```python
from build123d import *

# Parameters (mm, degrees)
SKETCH1_R           = 79.480373192
BOSS_EXTRUDE1_DEPTH = 10
BOSS_EXTRUDE2_DEPTH = 70
FILLET3_R           = 5
SKETCH7_R           = 2.5
CUT_EXTRUDE4_DEPTH  = 138.964703622
CUT_EXTRUDE6_DEPTH  = 2.5
FILLET5_RADIUS      = 20
FILLET5_LENGTH      = 10
CUT_EXTRUDE7_DEPTH  = 2.5


with BuildPart() as part:
    # Sketch1 → Boss-Extrude1 (new body)
    with BuildSketch(Plane.XY):
        Circle(SKETCH1_R)
    extrude(amount=BOSS_EXTRUDE1_DEPTH)

    # Sketch2 → Boss-Extrude2 (add)
    with BuildSketch(Plane.XY.offset(10)):
        Polygon((0, 0), (0, -20), (-10, -20), (-10, 20), (0, 20), align=None)
    extrude(amount=BOSS_EXTRUDE2_DEPTH)

    # Fillet3
    fillet3_edges = [part.edges().sort_by_distance(p)[0] for p in [
        (-5, 20, 10),
        (-10, 0, 10),
        (-5, -20, 10),
        (0, 0, 10),
    ]]
    fillet(fillet3_edges, radius=FILLET3_R)

    # Sketch7 → Cut-Extrude4 (cut, through all)
    with BuildSketch(Plane(origin=(0, 0, 0), x_dir=(0, 0, -1), z_dir=(1, 0, 0))):
        with Locations(Location((-60, 0, 0), (0, 0, 90))):
            Circle(SKETCH7_R)
    extrude(amount=-CUT_EXTRUDE4_DEPTH, mode=Mode.SUBTRACT)

    # Sketch9 → Cut-Extrude6 (cut)
    with BuildSketch(Plane(origin=(0, 0, 0), x_dir=(0, 0, -1), z_dir=(1, 0, 0))):
        with BuildLine():
            Line((-64.239646316, 13.566264372), (-64.768269058, 6.229526416))
            Line((-64.768269058, 6.229526416), (-71.988493293, 7.63506113))
            ThreePointArc((-71.988493293, 7.63506113), (-74.774746239, 6.140592282), (-73.868552739, 3.111490773))
            Line((-73.868552739, 3.111490773), (-67.779062658, -1.014678928))
            Line((-67.779062658, -1.014678928), (-72.606403544, -6.56480918))
            ThreePointArc((-72.606403544, -6.56480918), (-72.70528203, -9.725009436), (-69.628906423, -10.454773599))
            Line((-69.628906423, -10.454773599), (-63.010793601, -7.244205344))
            Line((-63.010793601, -7.244205344), (-60.617910251, -14.19987031))
            ThreePointArc((-60.617910251, -14.19987031), (-57.930535791, -15.865601718), (-55.760353684, -13.566264372))
            Line((-55.760353684, -13.566264372), (-55.231730942, -6.229526416))
            Line((-55.231730942, -6.229526416), (-48.011506707, -7.63506113))
            ThreePointArc((-48.011506707, -7.63506113), (-45.225253761, -6.140592282), (-46.131447261, -3.111490773))
            Line((-46.131447261, -3.111490773), (-52.220937342, 1.014678928))
            Line((-52.220937342, 1.014678928), (-47.393596456, 6.56480918))
            ThreePointArc((-47.393596456, 6.56480918), (-47.29471797, 9.725009436), (-50.371093577, 10.454773599))
            Line((-50.371093577, 10.454773599), (-56.989206399, 7.244205344))
            Line((-56.989206399, 7.244205344), (-59.382089749, 14.19987031))
            ThreePointArc((-59.382089749, 14.19987031), (-62.069464209, 15.865601718), (-64.239646316, 13.566264372))
        make_face()
    extrude(amount=-CUT_EXTRUDE6_DEPTH, mode=Mode.SUBTRACT)

    # Fillet5: full round fillet: the end face becomes a half cylinder, R = half its width
    fillet5_face = Plane((-5, 0, 80), x_dir=(-1, 0, 0), z_dir=(0, 0, 1))  # on the end face: x along it, z out of the body
    fillet5_slab = fillet5_face.offset(-FILLET5_RADIUS / 2) * Box(FILLET5_LENGTH, 2 * FILLET5_RADIUS, FILLET5_RADIUS, mode=Mode.PRIVATE)  # the body's end, R deep
    fillet5_round = Plane((-5, 0, 60), x_dir=(0, 0, 1), z_dir=(-1, 0, 0)) * Cylinder(FILLET5_RADIUS, FILLET5_LENGTH, mode=Mode.PRIVATE)  # its axis R under the face
    add(fillet5_slab - fillet5_round, mode=Mode.SUBTRACT)

    # Sketch4 → Cut-Extrude7 (cut)
    with BuildSketch(Plane(origin=(0, 0, 0), x_dir=(-1, 0, 0), z_dir=(0, 0, -1))):
        with BuildLine():
            Line((-9.121537298, 10.900260879), (-6.793934197, 3.922479738))
            Line((-6.793934197, 3.922479738), (-14.000671478, 2.449352582))
            ThreePointArc((-14.000671478, 2.449352582), (-16, 0), (-14.000671478, -2.449352582))
            Line((-14.000671478, -2.449352582), (-6.793934197, -3.922479738))
            Line((-6.793934197, -3.922479738), (-9.121537298, -10.900260879))
            ThreePointArc((-9.121537298, -10.900260879), (-8, -13.856406461), (-4.87913418, -13.349613461))
            Line((-4.87913418, -13.349613461), (0, -7.844959475))
            Line((0, -7.844959475), (4.87913418, -13.349613461))
            ThreePointArc((4.87913418, -13.349613461), (8, -13.856406461), (9.121537298, -10.900260879))
            Line((9.121537298, -10.900260879), (6.793934197, -3.922479738))
            Line((6.793934197, -3.922479738), (14.000671478, -2.449352582))
            ThreePointArc((14.000671478, -2.449352582), (16, 0), (14.000671478, 2.449352582))
            Line((14.000671478, 2.449352582), (6.793934197, 3.922479738))
            Line((6.793934197, 3.922479738), (9.121537298, 10.900260879))
            ThreePointArc((9.121537298, 10.900260879), (8, 13.856406461), (4.87913418, 13.349613461))
            Line((4.87913418, 13.349613461), (0, 7.844959475))
            Line((0, 7.844959475), (-4.87913418, 13.349613461))
            ThreePointArc((-4.87913418, 13.349613461), (-8, 13.856406461), (-9.121537298, 10.900260879))
        make_face()
    extrude(amount=-CUT_EXTRUDE7_DEPTH, mode=Mode.SUBTRACT)


solid = part.part
```
Part model, mm, in its own coordinate system. A direction names the side the tool comes from. Round coordinates to 2 decimals unless told otherwise and drop trailing zeros. Order: outer loops, then holes, each group sorted by start corner. A loop starts at its lowest first (then second) coordinate and runs counter-clockwise, first axis right, second up. Notation, with made-up numbers: M -10,-6 L 3,-6 A24 ccw 3,31 Z; hole C 0.25,16.25 d9. An arc over 180 degrees is marked long. Answer in a Markdown table with one row per item. Add a question column.
Q1. Wall check: L1, parallel to Z at x = -6.75, y = 0; L2, parallel to Y at x = -1.5, z = 51.5; L3, parallel to X at y = -19, z = 22.5. Give the ranges that are in metal, low to high. Write a range as from..to.
Q2. 3-axis set-ups, long thin cutter, end or side, ignore diameter. For faces 1 (the face through (-2.474, 10.636, 1.232)), 2 (the face through (-5, -20, 37)), 3 (the face through (-1.2, -3.8, 70.2)): which of +Z, -Z, +X, -X, +Y, -Y reach the whole face in a straight line?
Q3. Cut at B-B on y = 58. Give the cut face in (x, z).
Q4. Mould opens along Z. For faces 4 (the face through (-1.2, 3.8, 49.8)), 5 (the face through (-10, 0, 47)), 6 (the face through (-5, -22, 11)), 7 (the face through (0, 0, 2.5)) say: +Z half, -Z half, draft (parallel to the pull), parting line (faces both ways), or undercut.
Q5. Pin check, flat tips, straight feed: pin 1 (8 mm diameter, centred on x = -46, y = 50, fed in from +Z); pin 2 (1.5 mm diameter, centred on y = 13, z = 59, fed in from -X); pin 3 (8 mm diameter, centred on x = -3.5, y = 11.5, fed in from -Z); pin 4 (2 mm diameter, centred on y = -18, z = 9, fed in from +X). Stop position of each tip, or through.
Q6. Cut at A-A on z = 36.5. Give the cut face in (x, y), and give its area (3 significant figures).
Established:
| question | item | result |
|---|---|---|
| 1 | L1 | z = 2.5..57.5, 62.5..80 |
| 1 | L2 | y = -20..-6.96, 0.53..1.84, 9.91..20 |
| 1 | L3 | x = -10..0 |
| 2 | face 1 | -Z |
| 2 | face 2 | +Z, +X, -X, -Y |
| 2 | face 3 | +X |
| 3 | outline | M -54.34,0 L 54.34,0 L 54.34,10 L -54.34,10 Z |
| 4 | face 4 | undercut |
| 4 | face 5 | draft |
| 4 | face 6 | +Z half |
| 4 | face 7 | -Z half |
| 5 | pin 1 | stops at z = 10 |
| 5 | pin 2 | stops at x = -10 |
| 5 | pin 3 | stops at z = 0 |
| 5 | pin 4 | stops at x = 77.64 |
| 6 | outline | M -10,-20 L 0,-20 L 0,20 L -10,20 Z |
| 6 | area | 400 mm2 |
